from build123d import *

# Parameters (mm, degrees)
SKETCH2_W           = 15
SKETCH2_H           = 6
SKETCH2_W_2         = 2.5
SKETCH2_H_2         = 15
BOSS_EXTRUDE1_DEPTH = 3
CUT_EXTRUDE1_DEPTH  = 4


with BuildPart() as part:
    # Sketch2 → Boss-Extrude1 (new body)
    with BuildSketch(Plane.XY):
        Polygon((-22.073806452, 10.862903226), (-22.073806452, 7.862903226), (-32.073806452, 7.862903226), (-32.073806452, -17.137096774), (17.926193548, -17.137096774), (17.926193548, -12.137096774), (14.926193548, -12.137096774), (14.926193548, 2.862903226), (17.926193548, 2.862903226), (17.926193548, 7.862903226), (12.926193548, 7.862903226), (12.926193548, 10.862903226), (-2.073806452, 10.862903226), (-2.073806452, 7.862903226), (-7.073806452, 7.862903226), (-7.073806452, 10.862903226), align=None)
        with Locations((-19.573806452, -4.137096774)):
            Rectangle(SKETCH2_W, SKETCH2_H, mode=Mode.SUBTRACT)
        with Locations((-5.573806452, -3.653225806)):
            Rectangle(SKETCH2_W_2, SKETCH2_H_2, mode=Mode.SUBTRACT)
    extrude(amount=BOSS_EXTRUDE1_DEPTH)

    # Sketch4 → Cut-Extrude1 (cut, through all)
    with BuildSketch(Plane.XY.offset(3)):
        Polygon((-22.073806452, 1.862903226), (-22.073806452, 7.862903226), (-32.073806452, 7.862903226), (-32.073806452, 1.862903226), (-32.073806452, -17.137096774), (-22.073806452, -17.137096774), align=None)
    extrude(amount=-CUT_EXTRUDE1_DEPTH, mode=Mode.SUBTRACT)


solid = part.part
Could you check a few things on this model? Use its own coordinates, in mm. A direction names the side the tool comes from. Coordinates: 2 decimals unless noted, no trailing zeros. Order: outer loops, then holes, each group sorted by start corner. A loop starts at its lowest first (then second) coordinate and runs counter-clockwise, first axis right, second up. Notation, with made-up numbers: (11.25, 76) -> (30.25, 76) arc R27 ccw to (30.25, 101) -> close; hole circle Ø8 at (-37, 64). An arc over 180 degrees is marked (long way). One line per question, with ' | ' between items.
Q1. Imagine slicing it at A-A on y = -8.75. Please give me the cut outline in (x, z), and give its area (4 significant figures).
Return value:
outline: (-22.07, 0) -> (-6.82, 0) -> (-6.82, 3) -> (-22.07, 3) -> close; (-4.32, 0) -> (14.93, 0) -> (14.93, 3) -> (-4.32, 3) -> close | area: 103.5 mm²
Q2. Imagine slicing it at D-D on x = -3.5. Please give me the cut outline in (y, z).
Return value:
outline: (-17.14, 0) -> (7.86, 0) -> (7.86, 3) -> (-17.14, 3) -> close
Q3. If I drill on L1, parallel to Y at x = -19.5, z = 1.95; L2, parallel to X at y = 8.75, z = 0.25; L3, parallel to X at y = -1.5, z = 2.95, over which ranges is the centre line in solid material (lowest first)?
Return value:
L1: -17.14 to -7.14, -1.14 to 10.86 | L2: -22.07 to -7.07, -2.07 to 12.93 | L3: -12.07 to -6.82, -4.32 to 14.93
Q4. On a 3-axis mill with a long thin cutter (end or side, diameter ignored), from which of +Z, -Z, +X, -X, +Y, -Y can I reach the whole of each face in a straight line? I mean faces 1 (the face through (-17, -1.137, 1)), 2 (the face through (16, 2.863, 1)), 3 (the face through (-7.074, 9, 1)), 4 (the face through (-4.324, -4, 1)). Say none if no direction works.
Return value:
face 1: +Z, -Z, -X | face 2: +Z, -Z, +X | face 3: +Z, -Z, +Y | face 4: +Z, -Z
Q5. I'm going to push flat-ended pins straight in: P1, Ø0.9, axis at y = 9.5, z = 1.5, coming from the +X side; P2, Ø0.9, axis at y = -4.5, z = 1, coming from the -X side; P3, Ø1.5, axis at y = -1.5, z = 2, coming from the +X side; P4, Ø1, axis at x = -13.5, y = -2.5, coming from the +Z side. Where does each tip first touch, or does it pass through?
Return value:
P1: x = 12.93 | P2: x = -12.07 | P3: x = 14.93 | P4: through
Q6. Imagine slicing it at C-C on y = -2.25. Please give me the cut outline in (x, z).
Return value:
outline: (-12.07, 0) -> (-6.82, 0) -> (-6.82, 3) -> (-12.07, 3) -> close; (-4.32, 0) -> (14.93, 0) -> (14.93, 3) -> (-4.32, 3) -> close
Q7. Imagine slicing it at B-B on z = 0.85. Please give me the cut outline in (x, y).
Return value:
outline: (-22.07, -17.14) -> (17.93, -17.14) -> (17.93, -12.14) -> (14.93, -12.14) -> (14.93, 2.86) -> (17.93, 2.86) -> (17.93, 7.86) -> (12.93, 7.86) -> (12.93, 10.86) -> (-2.07, 10.86) -> (-2.07, 7.86) -> (-7.07, 7.86) -> (-7.07, 10.86) -> (-22.07, 10.86) -> (-22.07, -1.14) -> (-12.07, -1.14) -> (-12.07, -7.14) -> (-22.07, -7.14) -> close; hole (-6.82, -11.15) -> (-4.32, -11.15) -> (-4.32, 3.85) -> (-6.82, 3.85) -> close
Q8. Thinking about a two-plate mould opening in X: for faces 5 (the face through (-6, -11.153, 1)), 6 (the face through (-5, 7.863, 1)), 7 (the face through (-22.074, -12, 2)), 8 (the face through (-2, -3, 0)), which applies, pulls with the +X half, pulls with the -X half, needs draft (parallel to the pull), parting line crosses it, or undercut?
Return value:
face 5: undercut | face 6: undercut | face 7: pulls with the -X half | face 8: needs draft
